Autodesk Inventor part; units mm, degrees
ref_plane "YZ Plane" through (0, 0, 0) normal (1, 0, 0) x (0, 1, 0)
ref_plane "XZ Plane" through (0, 0, 0) normal (0, 1, 0) x (-1, 0, 0)
ref_plane "XY Plane" through (0, 0, 0) normal (0, 0, 1) x (1, 0, 0)
sketch "Sketch1" plane through (0, 0, 0) normal (0, 1, 0) x (-1, 0, 0)
  line L0 (127.5, -200) -> (-127.5, -200)
  line L1 (-127.5, -200) -> (-127.5, 200)
  line L2 (-127.5, 200) -> (127.5, 200)
  line L3 (127.5, 200) -> (127.5, -200)
  line L4 (127.5, -200) -> (-127.5, 200) construction
  line L5 (-127.5, -200) -> (127.5, 200) construction
  point P0 (0, 0)
  dimension "d0" = 255
  dimension "d1" = 400
extrude "base" add sketch "Sketch1" along normal blind 5
sketch "Sketch5" plane through (0, 5, 0) normal (0, 1, 0) x (1, 0, 0)
  line L0 (-127.5, -200) -> (127.5, -200)
  line L1 (-110, -200) -> (-90, -200)
  line L2 (-90, -200) -> (-90, -195)
  line L3 (-90, -195) -> (-110, -195)
  line L4 (-110, -195) -> (-110, -200)
  line L5 (-60, -200) -> (-40, -200)
  line L6 (-40, -200) -> (-40, -195)
  line L7 (-40, -195) -> (-60, -195)
  line L8 (-60, -195) -> (-60, -200)
  line L9 (-10, -200) -> (10, -200)
  line L10 (10, -200) -> (10, -195)
  line L11 (10, -195) -> (-10, -195)
  line L12 (-10, -195) -> (-10, -200)
  line L13 (40, -200) -> (60, -200)
  line L14 (60, -200) -> (60, -195)
  line L15 (60, -195) -> (40, -195)
  line L16 (40, -195) -> (40, -200)
  line L17 (90, -200) -> (110, -200)
  line L18 (110, -200) -> (110, -195)
  line L19 (110, -195) -> (90, -195)
  line L20 (90, -195) -> (90, -200)
  line L21 (-110, 200) -> (-110, 195)
  line L22 (-90, 200) -> (-110, 200)
  line L23 (-110, 195) -> (-90, 195)
  line L24 (-90, 195) -> (-90, 200)
  line L25 (-60, 200) -> (-60, 195)
  line L26 (-40, 200) -> (-60, 200)
  line L27 (-40, 195) -> (-40, 200)
  line L28 (-10, 200) -> (-10, 195)
  line L29 (10, 200) -> (-10, 200)
  line L30 (10, 195) -> (10, 200)
  line L31 (-10, 195) -> (10, 195)
  line L32 (-60, 195) -> (-40, 195)
  line L33 (40, 200) -> (40, 195)
  line L34 (40, 195) -> (60, 195)
  line L35 (60, 200) -> (40, 200)
  line L36 (60, 195) -> (60, 200)
  line L37 (90, 200) -> (90, 195)
  line L38 (90, 195) -> (110, 195)
  line L39 (110, 200) -> (90, 200)
  line L40 (110, 195) -> (110, 200)
  point P0 (0, 0)
  point P1 (90, -200)
  point P2 (110, -200)
  point P3 (-10, -200)
  point P4 (10, -200)
  point P5 (-60, -200)
  point P6 (-40, -200)
  point P7 (40, -200)
  point P8 (60, -200)
  dimension "d36" = 20
  dimension "d37" = 5
  dimension "d40" = 50
  dimension "d45" = 17.5
  dimension "d46" = 17.5
  dimension "d49" = 395
extrude "Extrusion4" cut sketch "Sketch5" against normal blind 5
sketch "Sketch8" plane through (0, 5, 0) normal (0, 1, 0) x (1, 0, 0)
  line L0 (-127.5, 200) -> (-127.5, -200)
  line L1 (-127.5, -145) -> (-122.5, -145)
  line L2 (-122.5, -145) -> (-122.5, -165)
  line L3 (-122.5, -165) -> (-127.5, -165)
  line L4 (-127.5, -165) -> (-127.5, -145)
  line L5 (-127.5, -95) -> (-122.5, -95)
  line L6 (-122.5, -95) -> (-122.5, -115)
  line L7 (-122.5, -115) -> (-127.5, -115)
  line L8 (-127.5, -115) -> (-127.5, -95)
  line L9 (-127.5, -45) -> (-122.5, -45)
  line L10 (-122.5, -45) -> (-122.5, -65)
  line L11 (-122.5, -65) -> (-127.5, -65)
  line L12 (-127.5, -65) -> (-127.5, -45)
  line L13 (-127.5, 5) -> (-122.5, 5)
  line L14 (-122.5, 5) -> (-122.5, -15)
  line L15 (-122.5, -15) -> (-127.5, -15)
  line L16 (-127.5, -15) -> (-127.5, 5)
  line L17 (-127.5, 55) -> (-122.5, 55)
  line L18 (-122.5, 55) -> (-122.5, 35)
  line L19 (-122.5, 35) -> (-127.5, 35)
  line L20 (-127.5, 35) -> (-127.5, 55)
  line L21 (-127.5, 105) -> (-122.5, 105)
  line L22 (-122.5, 105) -> (-122.5, 85)
  line L23 (-122.5, 85) -> (-127.5, 85)
  line L24 (-127.5, 85) -> (-127.5, 105)
  line L25 (-127.5, 155) -> (-122.5, 155)
  line L26 (-122.5, 155) -> (-122.5, 135)
  line L27 (-122.5, 135) -> (-127.5, 135)
  line L28 (-127.5, 135) -> (-127.5, 155)
  line L29 (0, 0) -> (0, -33.5633)
  line L30 (127.5, -145) -> (122.5, -145)
  line L31 (122.5, -145) -> (122.5, -165)
  line L32 (122.5, -165) -> (127.5, -165)
  line L33 (127.5, -165) -> (127.5, -145)
  line L34 (127.5, -95) -> (122.5, -95)
  line L35 (122.5, -95) -> (122.5, -115)
  line L36 (122.5, -115) -> (127.5, -115)
  line L37 (127.5, -115) -> (127.5, -95)
  line L38 (127.5, -45) -> (122.5, -45)
  line L39 (122.5, -45) -> (122.5, -65)
  line L40 (122.5, -65) -> (127.5, -65)
  line L41 (127.5, -65) -> (127.5, -45)
  line L42 (127.5, 5) -> (122.5, 5)
  line L43 (122.5, 5) -> (122.5, -15)
  line L44 (122.5, -15) -> (127.5, -15)
  line L45 (127.5, -15) -> (127.5, 5)
  line L46 (127.5, 55) -> (122.5, 55)
  line L47 (122.5, 55) -> (122.5, 35)
  line L48 (122.5, 35) -> (127.5, 35)
  line L49 (127.5, 35) -> (127.5, 55)
  line L50 (127.5, 105) -> (122.5, 105)
  line L51 (122.5, 105) -> (122.5, 85)
  line L52 (122.5, 85) -> (127.5, 85)
  line L53 (127.5, 85) -> (127.5, 105)
  line L54 (127.5, 155) -> (122.5, 155)
  line L55 (122.5, 155) -> (122.5, 135)
  line L56 (122.5, 135) -> (127.5, 135)
  line L57 (127.5, 135) -> (127.5, 155)
  dimension "d82" = 5
  dimension "d83" = 20
  dimension "d84" = 35
  dimension "d87" = 50
extrude "Extrusion7" cut sketch "Sketch8" against normal blind 5
properties part number "base inferior"
Design review of the part built by this model. Coordinates are the model's own, in mm. Round coordinates to 2 decimals unless told otherwise and drop trailing zeros. Order: outer loops, then holes, each group sorted by start corner. A loop starts at its lowest first (then second) coordinate and runs counter-clockwise, first axis right, second up. Notation, with made-up numbers: M 80,22 L 127,22 A10 cw 127,40 Z; hole C 82.5,63 d4. An arc over 180 degrees is marked long. Put each result on its own line as item: value.
Q1. Consider section B-B (x = -105.5). State the section outline as (y, z) points.
Reported:
outline: M 0,-195 L 5,-195 L 5,195 L 0,195 Z
Q2. Consider section A-A (z = -50). State the section outline as (x, y) points.
Reported:
outline: M -122.5,0 L 122.5,0 L 122.5,5 L -122.5,5 Z
Q3. Insertion check: pin 1 Ø2.5 at (y, z) = (2, 54) entering from +X; pin 2 Ø1.5 at (x, y) = (3, 1.5) entering from +Z; pin 3 Ø1.5 at (x, y) = (94.5, 4) entering from -Z. Each pin has a flat end and moves straight along its axis. Give the tip position at first contact, or say it passes through.
Reported:
pin 1: x = 122.5
pin 2: z = 195
pin 3: z = -195
Q4. To check wall thickness, follow line 1 (Z direction, x = -98.5, y = 1.35); line 2 (X direction, y = 0.35, z = 7.5). State the ranges of each line that lie inside material, in increasing order.
Reported:
line 1: -195 to 195
line 2: -122.5 to 122.5
